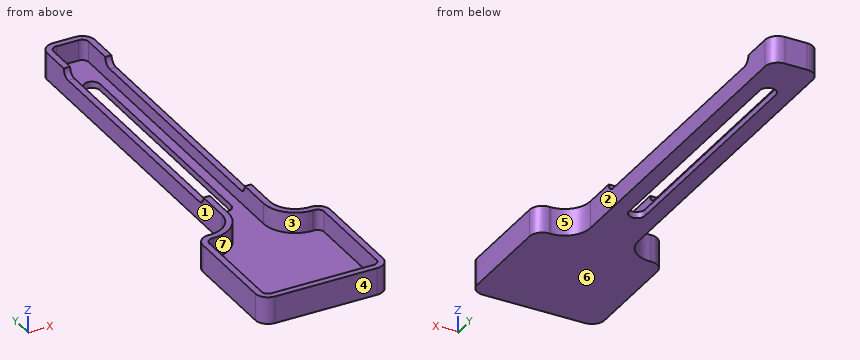
```python
from build123d import *

# Parameters (mm, degrees)
F3_DEPTH  = 8.5
F4_R      = 4
F5_R      = 8
F6_T      = -2
F8_DEPTH  = 2
F10_DEPTH = 15


with BuildPart() as f3:
    # F2 (on Top) → F3 (new body)
    with BuildSketch(Plane.XY):
        Polygon((-7.5, 19), (-20, 19), (-20, -19), (20, -19), (20, 19), (7.5, 19), (7.5, 131), (-7.5, 131), align=None)
    extrude(amount=F3_DEPTH)

    # F4
    f4_edges = [f3.edges().sort_by_distance(p)[0] for p in [
        (-20, 19, 4.25),
        (-20, -19, 4.25),
        (20, -19, 4.25),
        (20, 19, 4.25),
        (7.5, 131, 4.25),
        (-7.5, 131, 4.25),
    ]]
    fillet(f4_edges, radius=F4_R)

    # F5
    f5_edges = [f3.edges().sort_by_distance(p)[0] for p in [
        (7.5, 19, 4.25),
        (-7.5, 19, 4.25),
    ]]
    fillet(f5_edges, radius=F5_R)

    # F6
    f6_openings = [f3.faces().sort_by_distance(p)[0] for p in [
        (0, 39.190123, 8.5),
    ]]
    offset(amount=F6_T, openings=f6_openings)

    # F7 (on face) → F8 (cut, through all)
    with BuildSketch(Plane.XY.offset(2)):
        with BuildLine():
            ThreePointArc((2.5, 115), (0, 117.5), (-2.5, 115))
            Line((-2.5, 115), (-2.5, 40))
            ThreePointArc((-2.5, 40), (0, 37.5), (2.5, 40))
            Line((2.5, 40), (2.5, 115))
        make_face()
    extrude(amount=-F8_DEPTH, mode=Mode.SUBTRACT)

    # F9 (on face) → F10 (cut)
    with BuildSketch(Plane.YZ.offset(7.5)):
        with BuildLine():
            Line((115, 11), (40, 11))
            ThreePointArc((40, 11), (37.5, 8.5), (40, 6))
            Line((40, 6), (115, 6))
            ThreePointArc((115, 6), (117.5, 8.5), (115, 11))
        make_face()
    extrude(amount=-F10_DEPTH, mode=Mode.SUBTRACT)


solid = f3.part
```
CAD build for the part. Positions are in the model's coordinates, mm. Face numbers are marked on the shaded views. A direction names the side the tool comes from. Give positions to 0.01 mm unless a question says otherwise; leave off trailing zeros. Order: outer loops, then holes, each group sorted by start corner. A loop starts at its lowest first (then second) coordinate and runs counter-clockwise, first axis right, second up. Notation, with made-up numbers: M 50.25,49 L 96.25,49 A25 cw 96.25,70 Z; hole C 18,-17.75 d1. An arc over 180 degrees is marked long. Put each result on its own line as item: value. Start each with the question number.
(1) Saw through at D-D, the plane x = 10. Write the cut outline in (y, z), then the cut area to 3 significant figures.
(2) Drill centre lines: line 1 along X through (y, z) = (118.5, 3.5); line 2 along X through (y, z) = (-12, 6.25); line 3 along Y through (x, z) = (1.5, 8.25). Where is each one in solid material? Low to high.
(3) Flat gauge pins, fed straight in: pin 1 Ø5 at (y, z) = (86.5, 5.5) entering from -X; pin 2 Ø8 at (x, y) = (-14.5, 86) entering from +Z; pin 3 Ø0.6 at (x, z) = (16, 5) entering from +Y; pin 4 Ø1.5 at (x, z) = (-14, 7) entering from +Y. Where does each tip first touch, or does it go through?
(4) Saw through at B-B, the plane y = 54.5. Write the cut outline in (x, z), then the cut area to 3 significant figures.
(5) Saw through at A-A, the plane x = 0. Write the cut outline in (y, z).
(6) Which spindle directions (+Z, -Z, +X, -X, +Y, -Y) get a long thin tool onto all of the face, cutting with end or side? Do the marked faces 1, 2 and 3. Say none if no direction does.
(7) Mould opens along Y. For the marked faces 4, 5, 6 and 7 say: +Y half, -Y half, draft (parallel to the pull), parting line (faces both ways), or undercut.
Check result:
1. outline: M -19,0 L 21.19,0 L 21.19,8.5 L 18.65,8.5 L 18.65,2 L -17,2 L -17,8.5 L -19,8.5 Z
1. area: 110 mm2
2. line 1: x = -7.5 to -5.5, 5.5 to 7.5
2. line 2: x = -20 to -18, 18 to 20
2. line 3: y = -19 to -17, 129 to 131
3. pin 1: stops at x = -7.5
3. pin 2: passes through
3. pin 3: stops at y = 19
3. pin 4: stops at y = 19.32
4. outline: M -7.5,0 L -2.5,0 L -2.5,2 L -5.5,2 L -5.5,6 L -7.5,6 Z; M 2.5,0 L 7.5,0 L 7.5,6 L 5.5,6 L 5.5,2 L 2.5,2 Z
4. area: 36.0 mm2
5. outline: M -19,0 L 37.5,0 L 37.5,2 L -17,2 L -17,8.5 L -19,8.5 Z; M 117.5,0 L 131,0 L 131,8.5 L 129,8.5 L 129,2 L 117.5,2 Z
6. face 1: +Z, -Z, -X, +Y
6. face 2: +Z, -Z, +X, +Y
6. face 3: +Z
7. face 4: -Y half
7. face 5: +Y half
7. face 6: draft
7. face 7: undercut
